Source: CAD feature listing. Evaluate the final solid. Frame: model axes, mm. Coordinates: 2 decimals unless noted, no trailing zeros. Write each loop counter-clockwise with the first axis right and the second up, starting at its lowest first coordinate (ties: lowest second). Pieces come first, ordered by that corner, then holes. Notation, with made-up numbers: M 1.5,16 L 48.5,16 A14 cw 48.5,39 Z; hole C 42.25,16 d8. An arc over 180 degrees is marked long. Write item = value, one per line. Start each with the question number.
1. Line query: line 1 along X through (y, z) = (-4.75, -22); line 2 along X through (y, z) = (-6.25, -20); line 3 along Z through (x, y) = (19, -5.75). Output: solid intervals per line, ascending.
2. Section query C-C (x = 23.5). Output: boundary loops of the cut face in (y, z), then the cut area to 3 significant figures.
3. Pull-direction query (X, two-part tool) for faces 1 (the face through (-17.185, -3.757, -21.398)), 2 (the face through (34.644, -3.757, 28.135)), 3 (the face through (-34.096, -3.757, 30.325)), 4 (the face through (-1, 0, 10)); classes: pulls with the +X half, pulls with the -X half, needs draft (parallel to the pull), parting line crosses it, or undercut.
4. Section query B-B (z = 20). Output: boundary loops of the cut face in (x, y).
5. Section query A-A (y = -5.25). Output: boundary loops of the cut face in (x, z) (3 decimals).
```python
from build123d import *

# Parameters (mm, degrees)
F0_R     = 3.175
F1_DEPTH = 7.62


with BuildPart() as f1:
    # F0 (on Front) → F1 (new body)
    with BuildSketch(Plane.XZ):
        with BuildLine():
            Line((0, 69.85), (0, 101.6))
            ThreePointArc((0, 101.6), (-34.372719, 29.23068), (-38.1, -50.8))
            Line((-38.1, -50.8), (0, -50.8))
            Line((0, -50.8), (0, -4.064))
            ThreePointArc((0, -4.064), (-4.064, 0), (0, 4.064))
            Line((0, 4.064), (0, 57.15))
            ThreePointArc((0, 57.15), (-6.35, 63.5), (0, 69.85))
        make_face()
        with Locations((-20.213376, -22.352)):
            Circle(F0_R, mode=Mode.SUBTRACT)
        with BuildLine():
            ThreePointArc((38.1, -50.8), (34.372719, 29.23068), (0, 101.6))
            Line((0, 101.6), (0, 69.85))
            ThreePointArc((0, 69.85), (4.490128, 67.990128), (6.35, 63.5))
            ThreePointArc((6.35, 63.5), (4.490128, 59.009872), (0, 57.15))
            Line((0, 57.15), (0, 4.064))
            ThreePointArc((0, 4.064), (2.873682, 2.873682), (4.064, 0))
            ThreePointArc((4.064, 0), (2.873682, -2.873682), (0, -4.064))
            Line((0, -4.064), (0, -50.8))
            Line((0, -50.8), (38.1, -50.8))
        make_face()
    extrude(amount=F1_DEPTH)


solid = f1.part
```
Results are:
q1.line_1 = -40.43 to -23.37, -17.06 to 40.43
q1.line_2 = -40.44 to -22.35, -18.08 to 40.44
q1.line_3 = -50.8 to 70.8
q2.outline = M -7.62,-50.8 L 0,-50.8 L 0,61.17 L -7.62,61.17 Z
q2.area = 853 mm^2
q3.face_1 = undercut
q3.face_2 = pulls with the +X half
q3.face_3 = pulls with the -X half
q3.face_4 = needs draft
q4.outline = M -36.45,-7.62 L 36.45,-7.62 L 36.45,0 L -36.45,0 Z
q5.outline = M -38.1,-50.8 L 38.1,-50.8 A203.2 ccw 0,101.6 A203.2 ccw Z; hole C -20.213,-22.352 d6.35; hole C 0,63.5 d12.7; hole C 0,0 d8.128
